from build123d import *

# Parameters (mm, degrees)
EXTRUDE_THIN1_DEPTH = 36.25
SKETCH2_W           = 25
SKETCH2_H           = 72.5
BOSS_EXTRUDE1_DEPTH = 1.25
LPATTERN1_COUNT     = 5
LPATTERN1_PITCH     = 12.5


with BuildPart() as part:
    # Sketch1 → Extrude-Thin1 (new, symmetric)
    with BuildSketch(Plane(origin=(0, 0, 0), x_dir=(1, 0, 0), z_dir=(0, 1, 0))):
        with BuildLine():
            ThreePointArc((13.507557647, 21.03677462), (25, 0), (13.507557647, -21.03677462))
            Line((13.507557647, -21.03677462), (14.858313411, -23.140452082))
            ThreePointArc((14.858313411, -23.140452082), (27.5, 0), (14.858313411, 23.140452082))
            Line((14.858313411, 23.140452082), (13.507557647, 21.03677462))
        make_face()
    extrude(amount=EXTRUDE_THIN1_DEPTH, both=True)

    # Sketch2 → Boss-Extrude1 (add, symmetric)
    with BuildSketch(Plane.XY):
        with Locations((39, 0)):
            Rectangle(SKETCH2_W, SKETCH2_H)
    extrude(amount=BOSS_EXTRUDE1_DEPTH, both=True)

    # Sketch4 → Ø3.0mm Dowel Hole1 (revolve, cut)
    with BuildSketch(Plane(origin=(39.48578811, 26.25, 1.25), x_dir=(0, -1, 0), z_dir=(1, 0, 0))):
        Polygon((0, 0), (0, 2.5), (1.525, 2.5), (1.5, 2.475), (1.5, 0), align=None)
    f_3_0mm_dowel_hole1 = revolve(axis=Axis((39.48578811, 26.25, 7.6), (0, 0, -1)), mode=Mode.SUBTRACT)

    # LPattern1: Ø3.0mm Dowel Hole1 ×5
    with Locations(*[(0, -i * LPATTERN1_PITCH, 0) for i in range(1, LPATTERN1_COUNT)]):
        add(f_3_0mm_dowel_hole1, mode=Mode.SUBTRACT)


solid = part.part
Work out the finished part from the listing and answer in its coordinate system (mm). A direction names the side the tool comes from. Coordinates: 2 decimals unless noted, no trailing zeros. Loops run counter-clockwise (first coordinate to the right, second up) from the corner with the lowest first, then second, coordinate; pieces in that order, holes last. Notation, with made-up numbers: (88.5, 5) -> (132.5, 5) arc R19 cw to (132.5, 12) -> close; hole circle Ø4 at (57, 16). An arc over 180 degrees is marked (long way). Answer as CSV lines item,"result".
1) Flat-ended cylindrical pins translate along their axes: pin 1 (6 mm diameter, centred on x = 46, y = 15.5, fed in from +Z); pin 2 (5 mm diameter, centred on x = 39.49, y = 26.25, fed in from -Z); pin 3 (1.8 mm diameter, centred on x = 39.49, y = -11.25, fed in from -Z); pin 4 (6 mm diameter, centred on y = 26, z = 16, fed in from +X). Find the tip coordinate at first contact, or state that the pin passes through.
A:
pin 1,"stops at z = 1.25"
pin 2,"stops at z = -1.25"
pin 3,"passes through"
pin 4,"stops at x = 24.23"
2) The part is cut by section B-B (y = -16.5). Give the vertices of the cut face in (x, z), and give its area (3 significant figures).
A:
outline,"(13.51, -21.04) -> (14.86, -23.14) arc R27.5 ccw to (27.47, -1.25) -> (51.5, -1.25) -> (51.5, 1.25) -> (27.47, 1.25) arc R27.5 ccw to (14.86, 23.14) -> (13.51, 21.04) arc R25 cw to start"
area,"191 mm²"
3) Straight lines are drawn through the part: probe 1 along X at (y, z) = (26.25, -0.5) (3 decimals); probe 2 along Z at (x, y) = (42, 7.5); probe 3 along X at (y, z) = (13, 0). For each, find the intervals that lie inside material, in ascending order.
A:
probe 1,"x = 24.995 to 37.986, 40.986 to 51.5"
probe 2,"z = -1.25 to 1.25"
probe 3,"x = 25 to 38.19, 40.78 to 51.5"
4) The part is cut by section A-A (y = 13.75). Give the vertices of the cut face in (x, z) (3 decimals).
A:
outline,"(13.508, -21.037) -> (14.858, -23.14) arc R27.5 ccw to (27.472, -1.25) -> (37.961, -1.25) -> (37.986, -1.225) -> (37.986, 1.25) -> (27.472, 1.25) arc R27.5 ccw to (14.858, 23.14) -> (13.508, 21.037) arc R25 cw to start; (40.986, -1.225) -> (41.011, -1.25) -> (51.5, -1.25) -> (51.5, 1.25) -> (40.986, 1.25) -> close"
5) The part is cut by section C-C (x = 47). Give the vertices of the cut face in (y, z).
A:
outline,"(-36.25, -1.25) -> (36.25, -1.25) -> (36.25, 1.25) -> (-36.25, 1.25) -> close"
6) For a pull along Y with two mould halves and no side action, classify faces 1 (the face through (40.95, -23.42, 0.03)), 2 (the face through (25.4, 36.25, 0.1)), 3 (the face through (14.19, 0.51, -22.1)) as released by +Y, released by -Y, zero draft, split by the parting line, or undercut.
A:
face 1,"undercut"
face 2,"released by +Y"
face 3,"zero draft"
7) The part is cut by section D-D (z = 6.5). Give the vertices of the cut face in (x, y), and give its area (3 significant figures).
A:
outline,"(24.14, -36.25) -> (26.72, -36.25) -> (26.72, 36.25) -> (24.14, 36.25) -> close"
area,"187 mm²"
8) For faces 4 (the face through (40.95, -10.92, 0.03)), 5 (the face through (42, 1, -1.25)), 6 (the face through (42, 1, 1.25)), determine the directions among +Z, -Z, +X, -X, +Y, -Y from which every point of the face is accessible in a straight line to the end or side of a thin tool.
A:
face 4,"+Z, -Z"
face 5,"-Z, +X, +Y, -Y"
face 6,"+Z, +X, +Y, -Y"
